Design review of the part built by this model. Coordinates are the model's own, in mm. A direction names the side the tool comes from. Give positions to 0.01 mm unless a question says otherwise; leave off trailing zeros. Loops run counter-clockwise (first coordinate to the right, second up) from the corner with the lowest first, then second, coordinate; pieces in that order, holes last. Notation, with made-up numbers: M 76.5,53 L 90.5,53 A26 cw 90.5,79 Z; hole C -20,16 d4. An arc over 180 degrees is marked long. Use a Markdown table: item, result. Add a question column.
(1) Insertion check: pin 1 Ø12.5 at (x, y) = (-37.5, 136.5) entering from +Z; pin 2 Ø12.5 at (y, z) = (137.5, 22.5) entering from -X; pin 3 Ø7.5 at (y, z) = (137, 29) entering from +X. Each pin has a flat end and moves straight along its axis. Give the tip position at first contact, or say it passes through.
(2) For faces 4 (the face through (-890, -3, 25)), 5 (the face through (-1, 125, 11)), 6 (the face through (-1, 150, 11)), list the 3-axis set-ups (+Z, -Z, +X, -X, +Y, -Y) from which the entire face can be reached by the end or side of a thin tool; tool diameter is ignored.
(3) Add section A-A, the plane x = 0. Give the boundary of the cut face in (y, z).
(4) Add section B-B, the plane y = -212. Give the boundary of the cut face in (x, z), then the cut area to 3 significant figures.
(5) Draft analysis for pull direction X (two halves, no side actions). For faces 1 (the face through (-14, 250, -123)), 2 (the face through (790, -3, 25)), 3 (the face through (890, -3, 25)), state which applies: pulls with the +X half, pulls with the -X half, needs draft (parallel to the pull), parting line crosses it, or undercut.
(6) For probe 1 along X at (y, z) = (-196.5, 23); probe 2 along Z at (x, y) = (778.5, 117); probe 3 along Y at (x, z) = (31.5, 26.5), list the stretches that pass through material, from the lowest coordinate up.
(7) Add section C-C, the plane x = 690. Give the boundary of the cut face in (y, z).
```python
from build123d import *

# Parameters (mm, degrees)
F0_W     = 2000
F0_H     = 300
F1_DEPTH = 250
F2_W     = 100
F2_H     = 500
F3_DEPTH = 50
F5_START = -375
F5_DEPTH = 25


with BuildPart() as f1:
    # F0 (on Front) → F1 (new body, symmetric)
    with BuildSketch(Plane.XZ):
        with Locations((0, -150)):
            Rectangle(F0_W, F0_H)
    extrude(amount=F1_DEPTH, both=True)

    # F2 (on face) → F3 (join)
    with BuildSketch(Plane.XY):
        with Locations((840, 0)):
            Rectangle(F2_W, F2_H)
        with Locations((-840, 0)):
            Rectangle(F2_W, F2_H)
    extrude(amount=F3_DEPTH)

    # F4 (on face) → F5 (join)
    with BuildSketch(Plane.XZ.offset(250).offset(F5_START)):
        with BuildLine():
            ThreePointArc((25, 40), (0, 15), (-25, 40))
            Line((-25, 40), (-50, 40))
            Line((-50, 40), (-50, 0))
            Line((-50, 0), (50, 0))
            Line((50, 0), (50, 40))
            Line((50, 40), (25, 40))
        make_face()
    extrude(amount=-F5_DEPTH)


solid = f1.part
```
Established:
| question | item | result |
|---|---|---|
| 1 | pin 1 | z = 40 |
| 1 | pin 2 | x = -890 |
| 1 | pin 3 | x = 890 |
| 2 | face 4 | +Z, -X, +Y, -Y |
| 2 | face 5 | +Z, -Y |
| 2 | face 6 | +Z, +Y |
| 3 | outline | M -250,-300 L 250,-300 L 250,0 L 150,0 L 150,15 L 125,15 L 125,0 L -250,0 Z |
| 4 | outline | M -1000,-300 L 1000,-300 L 1000,0 L 890,0 L 890,50 L 790,50 L 790,0 L -790,0 L -790,50 L -890,50 L -890,0 L -1000,0 Z |
| 4 | area | 610,000 mm^2 |
| 5 | face 1 | needs draft |
| 5 | face 2 | undercut |
| 5 | face 3 | pulls with the +X half |
| 6 | probe 1 | -890 to -790, 790 to 890 |
| 6 | probe 2 | -300 to 0 |
| 6 | probe 3 | 125 to 150 |
| 7 | outline | M -250,-300 L 250,-300 L 250,0 L -250,0 Z |
